Source: CAD feature listing. Evaluate the final solid. Frame: model axes, mm. A direction names the side the tool comes from. Coordinates: 2 decimals unless noted, no trailing zeros. Write each loop counter-clockwise with the first axis right and the second up, starting at its lowest first coordinate (ties: lowest second). Pieces come first, ordered by that corner, then holes. Notation, with made-up numbers: (83, 73.25) - (130, 73.25) arc R16 ccw to (130, 99.25) - close; hole circle Ø2 at (-27, -36). An arc over 180 degrees is marked (long way). One line per question, with ' | ' between items. Start each with the question number.
Q1. Cut plane B-B, the plane y = -3. Return loops of the section in (x, z), plus the area to 3 significant figures.
Q2. Cut plane C-C, the plane x = 54.5. Return loops of the section in (y, z).
Q3. Contact query for flat-ended pins moving along their axis: P1, Ø10, axis at y = 20.5, z = 89.5, coming from the +X side; P2, Ø5, axis at y = 1.5, z = 30, coming from the -X side; P3, Ø1, axis at y = -13, z = 38.5, coming from the -X side. Output: stop coordinate, or through.
Q4. Line query: line 1 (Z direction, x = -33, y = 56.5); line 2 (Y direction, x = -2, z = 172); line 3 (Y direction, x = -26, z = 14). Output: solid intervals per line, ascending.
Q5. Cut plane D-D, the plane z = 107. Return loops of the section in (x, y), plus the area to 3 significant figures.
Q6. Access query for faces 1 (the face through (32.98, 56.21, 113.77)), 2 (the face through (-64.905, 38.08, 189.967)), 3 (the face through (-32.98, -56.21, 113.77)). Directions: +Z, -Z, +X, -X, +Y, -Y. A direction counts if a zero-diameter tool reaches every point of the face in a straight line with its end or side. Return the directions, or none.
Q7. Draft query along Z for faces 4 (the face through (-32.189, 56.664, 113.767)), 5 (the face through (-65.43, -37.17, 189.97)), 6 (the face through (-1, 1, 0)). Return one class per face: +Z half, -Z half, draft (parallel to the pull), parting line (faces both ways), or undercut.
Q8. Cut plane A-A, the plane z = 203. Return loops of the section in (x, y), plus the area to 3 significant figures.
```python
from build123d import *

# Parameters (mm, degrees)
F1_DEPTH = 76.2
F3_DEPTH = 76.2
F5_DEPTH = 76.2


with BuildPart() as f1:
    # F0 (on Top) → F1 (new body)
    with BuildSketch(Plane.XY):
        Polygon((43.789267, -75.609836), (87.374672, 0.1177), (43.585405, 75.727536), (-43.789267, 75.609836), (-87.374672, -0.1177), (-43.585405, -75.727536), align=None)
    extrude(amount=F1_DEPTH)

    # F2 (on face) → F3 (join)
    with BuildSketch(Plane.XY.offset(76.2)):
        Polygon((-0.082408, 75.248235), (-65.208088, 37.55275), (-65.125679, -37.695485), (0.082408, -75.248235), (65.208088, -37.55275), (65.125679, 37.695485), align=None)
    extrude(amount=F3_DEPTH)

    # F4 (on face) → F5 (join)
    with BuildSketch(Plane.XY.offset(152.4)):
        Polygon((43.526997, -75.200657), (86.889178, 0.095157), (43.362181, 75.295814), (-43.526997, 75.200657), (-86.889178, -0.095157), (-43.362181, -75.295814), align=None)
    extrude(amount=F5_DEPTH)


solid = f1.part
```
Reply:
1) outline: (-85.71, 0) - (85.58, 0) - (85.58, 76.2) - (65.17, 76.2) - (65.17, 152.4) - (85.11, 152.4) - (85.11, 228.6) - (-85.21, 228.6) - (-85.21, 152.4) - (-65.16, 152.4) - (-65.16, 76.2) - (-85.71, 76.2) - close | area: 36,000 mm^2
2) outline: (-57, 0) - (56.88, 0) - (56.88, 76.2) - (43.81, 76.2) - (43.81, 152.4) - (56.05, 152.4) - (56.05, 228.6) - (-56.15, 228.6) - (-56.15, 152.4) - (-43.75, 152.4) - (-43.75, 76.2) - (-57, 76.2) - close
3) P1: stops at x = 65.15 | P2: stops at x = -87.37 | P3: stops at x = -80.2
4) line 1: z = 0 to 76.2, 152.4 to 228.6 | line 2: y = -75.25 to 75.25 | line 3: y = -75.7 to 75.63
5) outline: (-65.21, 37.55) - (-65.13, -37.7) - (0.08, -75.25) - (65.21, -37.55) - (65.13, 37.7) - (-0.08, 75.25) - close | area: 14,700 mm^2
6) face 1: +X, +Y | face 2: +Z, -X, +Y | face 3: -X, -Y
7) face 4: undercut | face 5: draft | face 6: -Z half
8) outline: (-86.89, -0.1) - (-43.36, -75.3) - (43.53, -75.2) - (86.89, 0.1) - (43.36, 75.3) - (-43.53, 75.2) - close | area: 19,600 mm^2
